Could you check a few things on this model? Use its own coordinates, in mm. Round coordinates to 2 decimals unless told otherwise and drop trailing zeros. Use CSV: the item, a comma, the result in double quotes. Start each with the question number.
```python
from build123d import *

# Parameters (mm, degrees)
F0_R     = 2.54
F1_DEPTH = 2.54


with BuildPart() as f1:
    # F0 (on Top) → F1 (new body)
    with BuildSketch(Plane.XY):
        with BuildLine():
            Line((-13.72965, -6.211935), (-10.352021, -6.211935))
            Line((-10.352021, -6.211935), (-7.658862, -6.211935))
            Line((-7.658862, -6.211935), (-2.500108, -6.211935))
            Line((-2.500108, -6.211935), (0.098243, -6.211935))
            Line((0.098243, -6.211935), (4.492023, -6.211935))
            Line((4.492023, -6.211935), (5.238309, -6.211935))
            Line((5.238309, -6.211935), (9.521089, -6.211935))
            Line((9.521089, -6.211935), (10.040419, -6.211935))
            Line((10.040419, -6.211935), (15.077152, -6.211935))
            Line((15.077152, -6.211935), (15.077152, -5.268871))
            Line((15.077152, -5.268871), (16.105427, -6.165902))
            Line((16.105427, -6.165902), (20.595906, -6.165902))
            Line((20.595906, -6.165902), (22.804618, -3.994572))
            Line((22.804618, -3.994572), (22.804618, -3.312337))
            ThreePointArc((22.804618, -3.312337), (31.332733, 0.11279), (22.656238, 3.142425))
            Line((22.656238, 3.142425), (22.656238, 4.226365))
            Line((22.656238, 4.226365), (22.302699, 4.611585))
            Line((22.302699, 4.611585), (20.876208, 6.165907))
            Line((20.876208, 6.165907), (15.069485, 6.165907))
            Line((15.069485, 6.165907), (10.040419, 6.165907))
            Line((10.040419, 6.165907), (9.521089, 6.165907))
            Line((9.521089, 6.165907), (5.238309, 6.165907))
            Line((5.238309, 6.165907), (4.492023, 6.165907))
            Line((4.492023, 6.165907), (1.025901, 6.165907))
            Line((1.025901, 6.165907), (-3.409077, 6.165907))
            Line((-3.409077, 6.165907), (-6.900202, 6.165907))
            Line((-6.900202, 6.165907), (-7.658862, 6.165907))
            Line((-7.658862, 6.165907), (-12.207904, 6.165907))
            Line((-12.207904, 6.165907), (-13.72965, 6.165907))
            Line((-13.72965, 6.165907), (-15.919671, 6.165907))
            Line((-15.919671, 6.165907), (-17.367226, 6.165907))
            Line((-17.367226, 6.165907), (-22.804618, 6.165907))
            Line((-22.804618, 6.165907), (-22.804618, 2.881158))
            Line((-22.804618, 2.881158), (-21.560945, 2.881158))
            Line((-21.560945, 2.881158), (-19.33411, -6.211935))
            Line((-19.33411, -6.211935), (-15.919671, -6.211935))
            Line((-15.919671, -6.211935), (-14.843066, -1.776392))
            Line((-14.843066, -1.776392), (-13.72965, -6.211935))
        make_face()
        Polygon((-11.094488, 5.107989), (-7.995496, 5.107989), (-7.995496, 3.976453), (-8.904465, 3.976453), (-11.206055, -5.13533), (-13.135563, -5.13533), (-14.824377, 1.730931), (-16.550569, -5.13533), (-18.480642, -5.13533), (-20.762977, 3.976453), (-21.691201, 3.976453), (-21.691201, 5.107989), (-18.480642, 5.107989), (-18.480642, 3.976453), (-19.408301, 3.976453), (-17.367226, -3.873531), (-15.158514, 5.107989), (-14.490804, 5.107989), (-12.300784, -3.873531), (-10.259141, 3.976453), (-11.094488, 3.976453), align=None, mode=Mode.SUBTRACT)
        Polygon((1.58261, 5.107989), (4.143582, 5.107989), (4.143582, 3.976453), (3.308802, 3.976453), (3.308802, -4.040601), (4.143582, -4.040601), (4.143582, -5.13533), (1.19297, -5.13533), (1.19297, -4.040601), (2.046439, -4.040601), (2.046439, 3.753313), (-0.885484, -1.219681), (-1.535071, -1.219681), (-4.466992, 3.827508), (-4.466992, -4.040601), (-3.594835, -4.040601), (-3.594835, -5.13533), (-6.564135, -5.13533), (-6.564135, -4.040601), (-5.710667, -4.040601), (-5.710667, 3.976453), (-6.564135, 3.976453), (-6.564135, 5.107989), (-3.910285, 5.107989), (-1.200932, 0.431753), align=None, mode=Mode.SUBTRACT)
        Polygon((11.135711, 5.107989), (13.974756, 5.107989), (13.974756, 3.976453), (13.121286, 3.976453), (13.121286, -4.021916), (13.974756, -4.021916), (13.974756, -5.13533), (11.135711, -5.13533), (11.135711, -4.021916), (11.618231, -4.021916), (11.618231, -0.440402), (7.943841, -0.440402), (7.943841, -4.021916), (8.40767, -4.021916), (8.40767, -5.13533), (5.735131, -5.13533), (5.735131, -4.021916), (6.44022, -4.021916), (6.44022, 3.976453), (5.735131, 3.976453), (5.735131, 5.107989), (8.40767, 5.107989), (8.40767, 3.976453), (7.943841, 3.976453), (7.943841, 0.691705), (11.618231, 0.691705), (11.618231, 3.976453), (11.135711, 3.976453), align=None, mode=Mode.SUBTRACT)
        Polygon((20.633285, 0.811923), (21.728014, -0.283368), (21.728014, -3.512052), (20.076579, -5.089298), (16.624759, -5.089298), (15.065635, -3.512052), (15.065635, -2.751466), (16.531877, -2.751466), (16.531877, -3.270793), (17.236968, -3.994572), (19.48249, -3.994572), (20.224959, -3.270793), (20.224959, -0.598818), (19.835318, -0.171801), (16.197742, -0.171801), (15.065635, 0.978994), (15.065635, 3.614156), (16.624759, 5.154023), (20.224959, 5.154023), (21.728014, 3.614156), (21.728014, 3.150327), (20.224959, 3.150327), (20.224959, 3.335517), (19.575371, 4.022482), (17.236968, 4.022482), (16.531877, 3.335517), (16.531877, 1.238374), (16.958896, 0.811923), align=None, mode=Mode.SUBTRACT)
        with Locations((26.426162, 0)):
            Circle(F0_R, mode=Mode.SUBTRACT)
    extrude(amount=F1_DEPTH)


solid = f1.part
```
1. Suppose I cut it at A-A (z = 2.15). State how many separate pieces and enclosed holes the cut face has, then the cut area to 3 significant figures.
2. We'd pull the mould along X, two halves only. Please class faces 1 (the face through (4, 0, 0)), 2 (the face through (-22.805, 5, 1)), 3 (the face through (3, 5.108, 1)): pulls with the +X half, pulls with the -X half, needs draft (parallel to the pull), parting line crosses it, or undercut.
3. Will these pins go through, and if not, where does the flat tip stop? pin 1 (0.5 mm diameter, centred on y = -3.5, z = 0.5, fed in from +X); pin 2 (1.5 mm diameter, centred on y = 4.5, z = 1.5, fed in from +X); pin 3 (0.6 mm diameter, centred on x = -22, z = 1.5, fed in from -Y); pin 4 (3 mm diameter, centred on x = -6.5, y = -3.5, fed in from -Z).
4. If I drill on L1, parallel to Y at x = 8, z = 2.25; L2, parallel to Y at x = 9.5, z = 0.5; L3, parallel to Y at x = 21.5, z = 1.2, over which ranges is the centre line in solid material (lowest first)?
Geometry check:
1,separate pieces,"1"
1,enclosed holes,"5"
1,area,"414 mm²"
2,face 1,"needs draft"
2,face 2,"pulls with the -X half"
2,face 3,"undercut"
3,pin 1,"stops at x = 30.1"
3,pin 2,"stops at x = 29.59"
3,pin 3,"stops at y = 2.88"
3,pin 4,"stops at z = 0"
4,L1,"y = -6.21 to -5.14, -4.02 to -0.44, 0.69 to 3.98, 5.11 to 6.17"
4,L2,"y = -6.21 to -0.44, 0.69 to 6.17"
4,L3,"y = -5.28 to -3.73, -0.06 to 3.15, 3.85 to 5.49"
